Check sheet for the modelled part. Datum: model origin and axes. Units: mm. A direction names the side the tool comes from. Coordinates: 2 decimals unless noted, no trailing zeros. Loops run counter-clockwise (first coordinate to the right, second up) from the corner with the lowest first, then second, coordinate; pieces in that order, holes last. Notation, with made-up numbers: (33.25, 72) -> (42.25, 72) arc R17 ccw to (42.25, 77) -> close; hole circle Ø9 at (-0.75, 65.25). An arc over 180 degrees is marked (long way). Use one line per item in the form item = value.
from build123d import *

# Parameters (mm, degrees)
EXTRUS_O1_START          = -8.5
EXTRUS_O1_OUTLINE_R      = 3.5
EXTRUS_O1_DEPTH          = 8.5
FILETE1_R                = 5
CIRPATTERN1_COUNT        = 3
FILETE1_OF_CIRPATTERN1_R = 5
ESBO_O3_R                = 48.5
ESBO_O3_R_2              = 22.5
CORTE_EXTRUS_O1_DEPTH    = 21
ESBO_O4_R                = 3.5
CORTE_EXTRUS_O2_DEPTH    = 102.505753245


# Read off the part's stored shape, not the designer's step: Extrusão1
with BuildPart() as part:
    # Esboço1 → Revolução1 (revolve)
    with BuildSketch(Plane.XY, mode=Mode.PRIVATE) as revolu_o1_sk:
        Polygon((0, 17.5), (29, 17.5), (29, 50), (24, 50), (24, 53.5), (0, 53.5), align=None)
    revolve(revolu_o1_sk.sketch.rotate(Axis((0, 0, 0), (1, 0, 0)), 90), axis=Axis((0, 0, 0), (1, 0, 0)))

    # Extrusão1 outline → Extrusão1 (add)
    with BuildSketch(Plane(origin=(24, 0, 0), x_dir=(0, 0, -1), z_dir=(1, 0, 0)).offset(EXTRUS_O1_START)):
        with BuildLine():
            Line((-7.627068165, 67.414164927), (-12.499978821, 52.019232304))
            ThreePointArc((-12.499978821, 52.019232304), (1.2458e-05, 53.5), (12.500003048, 52.019226482))
            Line((12.500003048, 52.019226482), (7.627010883, 67.414196325))
            ThreePointArc((7.627010883, 67.414196325), (-4.0138e-05, 73), (-7.627068165, 67.414164927))
        make_face()
        with Locations((-2.3672e-05, 65)):
            Circle(EXTRUS_O1_OUTLINE_R, mode=Mode.SUBTRACT)
    extrus_o1 = extrude(amount=EXTRUS_O1_DEPTH)

    # Filete1
    filete1_edges = [part.edges().sort_by_distance(p)[0] for p in [
        (19.75, 52.019232304, 12.499978821),
        (19.75, 52.019226482, -12.500003048),
    ]]
    fillet(filete1_edges, radius=FILETE1_R)

    # CirPattern1: Extrusão1 ×3 about axis
    cirpattern1_axis = Axis((0, 0, 0), (1, 0, 0))
    for i in range(1, CIRPATTERN1_COUNT):
        add(extrus_o1.rotate(cirpattern1_axis, i * 360 / CIRPATTERN1_COUNT))

    # Filete1 of CirPattern1
    filete1_of_cirpattern1_edges = [part.edges().sort_by_distance(p)[0] for p in [
        (19.75, -36.834915358, 38.79998725),
        (19.75, -15.184293054, 51.299973143),
        (19.75, -15.184316946, -51.299966071),
        (19.75, -36.834933428, -38.799970095),
    ]]
    fillet(filete1_of_cirpattern1_edges, radius=FILETE1_OF_CIRPATTERN1_R)

    # Esboço3 → Corte-extrusão1 (cut)
    with BuildSketch(Plane.ZY):
        Circle(ESBO_O3_R)
        Circle(ESBO_O3_R_2, mode=Mode.SUBTRACT)
    extrude(amount=-CORTE_EXTRUS_O1_DEPTH, mode=Mode.SUBTRACT)

    # Esboço4 → Corte-extrusão2 (cut, through all)
    with BuildSketch(Plane(origin=(29, 0, 0), x_dir=(0, 0, -1), z_dir=(1, 0, 0))):
        with Locations((-19.29163941, -37.5000205)):
            Circle(ESBO_O4_R)
    extrude(amount=-CORTE_EXTRUS_O2_DEPTH, mode=Mode.SUBTRACT)


solid = part.part
(1) Mould release check, pull along Y, two halves, no side actions. Record for faces 4 (the cylindrical face through (19.69, -36.62, -63.15)), 5 (the cylindrical face through (19.69, -34.63, -53.514)), 6 (the cylindrical face through (14.703, 17.084, -3.794)), 7 (the flat face through (15.5, -30, 52)): +Y half, -Y half, draft (parallel to the pull), parting line (faces both ways), or undercut.
Established:
face_4 = parting line
face_5 = undercut
face_6 = undercut
face_7 = draft
(2) Section check B-B, the plane y = 0. Record the boundary of the cut face in (x, z), plus the area to 3 significant figures.
Established:
outline = (0, -53.5) -> (24, -53.5) -> (24, -50) -> (29, -50) -> (29, -17.5) -> (0, -17.5) -> (0, -22.5) -> (21, -22.5) -> (21, -48.5) -> (0, -48.5) -> close; (0, 17.5) -> (29, 17.5) -> (29, 50) -> (24, 50) -> (24, 53.5) -> (0, 53.5) -> (0, 48.5) -> (21, 48.5) -> (21, 22.5) -> (0, 22.5) -> close
area = 961 mm²
(3) Go/stop test with flat-tipped pins: P1, Ø10, axis at x = 24, y = -18, coming from the +Z side; P2, Ø5, axis at x = 16, z = 21.5, coming from the -Y side; P3, Ø6.5, axis at y = -32.5, z = -56.29, coming from the +X side; P4, Ø6, axis at x = 18.5, z = -35, coming from the +Y side. Record where each tip stops, or that it passes through.
Established:
P1 = 58.45
P2 = -50.01
P3 = through
P4 = 42.87
(4) Section check D-D, the plane z = -24.5. Record the boundary of the cut face in (x, y), plus the area to 3 significant figures.
Established:
outline = (0, -47.56) -> (24, -47.56) -> (24, -43.59) -> (29, -43.59) -> (29, 43.59) -> (24, 43.59) -> (24, 47.56) -> (0, 47.56) -> (0, 41.86) -> (21, 41.86) -> (21, -41.86) -> (0, -41.86) -> close
area = 961 mm²
(5) Section check A-A, the plane z = 0. Record the boundary of the cut face in (x, y).
Established:
outline = (0, -53.5) -> (24, -53.5) -> (24, -50) -> (29, -50) -> (29, -17.5) -> (0, -17.5) -> (0, -22.5) -> (21, -22.5) -> (21, -48.5) -> (0, -48.5) -> close; (0, 17.5) -> (29, 17.5) -> (29, 50) -> (24, 50) -> (24, 61.5) -> (15.5, 61.5) -> (15.5, 53.5) -> (0, 53.5) -> (0, 48.5) -> (21, 48.5) -> (21, 22.5) -> (0, 22.5) -> close; (15.5, 68.5) -> (24, 68.5) -> (24, 73) -> (15.5, 73) -> close
(6) Scan lines: line 1 along Y through (x, z) = (13, 0); line 2 along Z through (x, y) = (19.5, 2); line 3 along Y through (x, z) = (22, 0). Record each from-to range of solid material in increasing order.
Established:
line_1 = -53.5 to -48.5, -22.5 to -17.5, 17.5 to 22.5, 48.5 to 53.5
line_2 = -53.46 to -48.46, -22.41 to -17.39, 17.39 to 22.41, 48.46 to 53.46
line_3 = -53.5 to -17.5, 17.5 to 61.5, 68.5 to 73
(7) Tool access check on faces 1 (the flat face through (15.5, -30, -52)), 2 (the cylindrical face through (10.353, -19.961, 10.382)), 3 (the flat face through (24, -37, 34)). Record the directions out of +Z, -Z, +X, -X, +Y, -Y that give a thin tool (end or side, any length) a straight path to the whole face; none if there is none.
Established:
face_1 = -Z, -X, -Y
face_2 = -X
face_3 = +X
(8) Section check C-C, the plane x = 3. Record the boundary of the cut face in (y, z).
Established:
outline = circle Ø107 at (0, 0); circle Ø45 at (0, 0); hole circle Ø97 at (0, 0); hole circle Ø35 at (0, 0)
